Source: CAD feature listing. Evaluate the final solid. Frame: model axes, mm. Give positions to 0.01 mm unless a question says otherwise; leave off trailing zeros. Order: outer loops, then holes, each group sorted by start corner. A loop starts at its lowest first (then second) coordinate and runs counter-clockwise, first axis right, second up. Notation, with made-up numbers: (28, -11) -> (84, -11) arc R14 cw to (84, -4) -> close; hole circle Ø7 at (23, 68). An arc over 180 degrees is marked (long way). Answer in a Markdown table with one row per item.
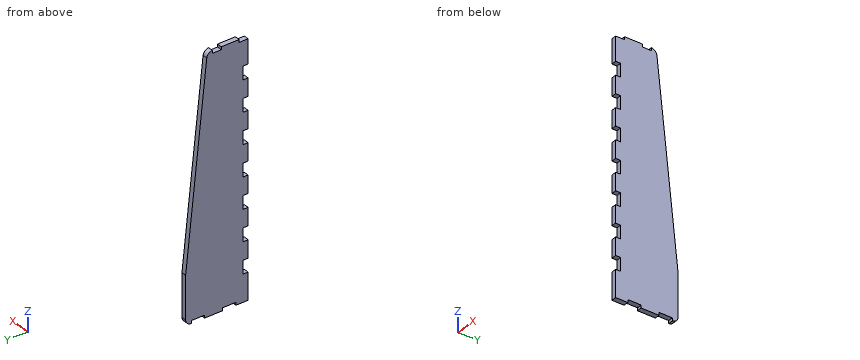
```python
from build123d import *

# Parameters (mm, degrees)
BOSS_EXTRUDE1_DEPTH = 5.588


with BuildPart() as part:
    # Sketch26 → Boss-Extrude1 (new body)
    with BuildSketch(Plane(origin=(0, 0, 0), x_dir=(0, 0, -1), z_dir=(1, 0, 0))):
        with BuildLine():
            Line((-3.175, -205.30682867), (-33.668926811, -205.30682867))
            Line((-33.668926811, -205.30682867), (-33.668926811, -199.71882867))
            Line((-33.668926811, -199.71882867), (-48.668926811, -199.71882867))
            Line((-48.668926811, -199.71882867), (-48.668926811, -205.30682867))
            Line((-48.668926811, -205.30682867), (-68.668926811, -205.30682867))
            Line((-68.668926811, -205.30682867), (-68.668926811, -199.71882867))
            Line((-68.668926811, -199.71882867), (-83.668926811, -199.71882867))
            Line((-83.668926811, -199.71882867), (-83.668926811, -205.30682867))
            Line((-83.668926811, -205.30682867), (-103.668926811, -205.30682867))
            Line((-103.668926811, -205.30682867), (-103.668926811, -199.71882867))
            Line((-103.668926811, -199.71882867), (-118.668926811, -199.71882867))
            Line((-118.668926811, -199.71882867), (-118.668926811, -205.30682867))
            Line((-118.668926811, -205.30682867), (-138.668926811, -205.30682867))
            Line((-138.668926811, -205.30682867), (-138.668926811, -199.71882867))
            Line((-138.668926811, -199.71882867), (-153.668926811, -199.71882867))
            Line((-153.668926811, -199.71882867), (-153.668926811, -205.30682867))
            Line((-153.668926811, -205.30682867), (-173.668926811, -205.30682867))
            Line((-173.668926811, -205.30682867), (-173.668926811, -199.71882867))
            Line((-173.668926811, -199.71882867), (-188.668926811, -199.71882867))
            Line((-188.668926811, -199.71882867), (-188.668926811, -205.30682867))
            Line((-188.668926811, -205.30682867), (-208.668926811, -205.30682867))
            Line((-208.668926811, -205.30682867), (-208.668926811, -199.71882867))
            Line((-208.668926811, -199.71882867), (-223.668926811, -199.71882867))
            Line((-223.668926811, -199.71882867), (-223.668926811, -205.30682867))
            Line((-223.668926811, -205.30682867), (-243.668926811, -205.30682867))
            Line((-243.668926811, -205.30682867), (-243.668926811, -199.71882867))
            Line((-243.668926811, -199.71882867), (-258.668926811, -199.71882867))
            Line((-258.668926811, -199.71882867), (-258.668926811, -205.30682867))
            Line((-258.668926811, -205.30682867), (-285.987853622, -205.30682867))
            Line((-285.987853622, -205.30682867), (-285.987853622, -195.30682867))
            Line((-285.987853622, -195.30682867), (-289.162853622, -195.30682867))
            Line((-289.162853622, -195.30682867), (-289.162853622, -175.30682867))
            Line((-289.162853622, -175.30682867), (-285.987853622, -175.30682867))
            Line((-285.987853622, -175.30682867), (-285.987853622, -165.30682867))
            Line((-285.987853622, -165.30682867), (-289.162853622, -165.30682867))
            ThreePointArc((-289.162853622, -165.30682867), (-287.531823263, -161.057849319), (-283.476609363, -158.991614634))
            Line((-283.476609363, -158.991614634), (-57.959024207, -135.288761307))
            ThreePointArc((-57.959024207, -135.288761307), (-57.802446686, -135.276438389), (-57.645438817, -135.272326993))
            Line((-57.645438817, -135.272326993), (-9.525, -135.272326993))
            ThreePointArc((-9.525, -135.272326993), (-5.034871939, -137.132198933), (-3.175, -141.622326993))
            Line((-3.175, -141.622326993), (-6.35, -141.622326993))
            Line((-6.35, -141.622326993), (-6.35, -156.622326993))
            Line((-6.35, -156.622326993), (-3.175, -156.622326993))
            Line((-3.175, -156.622326993), (-3.175, -176.622326993))
            Line((-3.175, -176.622326993), (-6.35, -176.622326993))
            Line((-6.35, -176.622326993), (-6.35, -191.622326993))
            Line((-6.35, -191.622326993), (-3.175, -191.622326993))
            Line((-3.175, -191.622326993), (-3.175, -205.30682867))
        make_face()
    extrude(amount=BOSS_EXTRUDE1_DEPTH)


solid = part.part
```
(1) Ray query, probe 1 along Z at (x, y) = (1.25, -177.5); probe 2 along Z at (x, y) = (2.1, -170) (3 decimals); probe 3 along Y at (x, z) = (1.4, 36). Return the intervals inside material, ascending.
A:
| item | result |
|---|---|
| probe 1 | z = 6.35 to 289.16 |
| probe 2 | z = 3.175 to 285.988 |
| probe 3 | y = -199.72 to -135.27 |
(2) First-contact query: pin 1 Ø1.6 at (x, z) = (3.5, 4.5) entering from +Y; pin 2 Ø3 at (x, y) = (2, -204) entering from +Z; pin 3 Ø1.5 at (x, y) = (4.5, -149) entering from -Z. Flat tips, straight axial feed; report the tip coordinate or a pass-through.
A:
| item | result |
|---|---|
| pin 1 | stops at y = -136.88 |
| pin 2 | stops at z = 285.99 |
| pin 3 | stops at z = 6.35 |
(3) Section query A-A (z = 143). Return the cut outline in (x, y), plus the area to 3 significant figures.
A:
| item | result |
|---|---|
| outline | (0, -199.72) -> (5.59, -199.72) -> (5.59, -144.23) -> (0, -144.23) -> close |
| area | 310 mm^2 |
(4) Section query B-B (y = -149). Return the cut outline in (x, z).
A:
| item | result |
|---|---|
| outline | (0, 6.35) -> (5.59, 6.35) -> (5.59, 188.41) -> (0, 188.41) -> close |
